```python
from build123d import *

# Parameters (mm, degrees)
F3_T     = -2.54
F5_D     = 7.62
F5_DEPTH = 38.101


# Not quite as in the source:
# - a feature of the source that left no trace in its solid (it failed there, or was rolled back) is left out


with BuildPart() as f1:
    # F0 (on Front) → F1 (revolve)
    with BuildSketch(Plane.XZ):
        Polygon((0, 0), (0, 63.5), (-38.1, 63.5), (-26.903236725, 0), align=None)
    revolve(axis=Axis((0, 0, 31.75), (0, 0, 1)))

    # F3
    f3_openings = [f1.faces().sort_by_distance(p)[0] for p in [
        (0, 0, 63.5),
    ]]
    offset(amount=F3_T, openings=f3_openings)

    # F5 (through all, one way)
    with BuildSketch(Plane.YZ):
        with Locations((0, 12.7)):
            Circle(F5_D / 2)
    extrude(amount=-F5_DEPTH, mode=Mode.SUBTRACT)


solid = f1.part
```
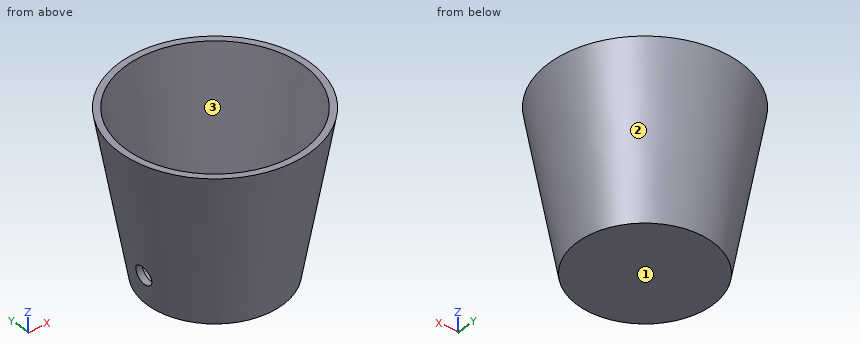
Here's how the part is built. I have some questions about the finished solid (model axes, mm). Face numbers are marked on the shaded views. Give positions to 0.01 mm unless a question says otherwise; leave off trailing zeros. Order: outer loops, then holes, each group sorted by start corner. A loop starts at its lowest first (then second) coordinate and runs counter-clockwise, first axis right, second up. Notation, with made-up numbers: (46, 62) - (61, 62) arc R7 ccw to (61, 70) - close; hole circle Ø11 at (53.25, -21.75). An arc over 180 degrees is marked (long way). Answer as a JSON object with one key per item and string values. Group by question number.
Item 1: If we section it at C-C on z = 21: Please give me the cut outline in (x, y).
Item 2: Please list where these lines run through material, in increasing order: probe 1 along Z at (x, y) = (-26.65, 0); probe 2 along Z at (x, y) = (-6, 2.5); probe 3 along Y at (x, z) = (24.5, 60.5).
Item 3: If we section it at B-B on z = 7.5: Please give me the cut outline in (x, y), and give its area (3 significant figures).
Item 4: If we mould it in two halves opening along X, with no side actions, what happens to the marked faces 1, 2 and 3? For each: pulls with the +X half, pulls with the -X half, needs draft (parallel to the pull), parting line crosses it, or undercut.
Item 5: For P1, Ø5, axis at y = -13, z = 26.5, coming from the +X side; P2, Ø12, axis at y = 5, z = 30, coming from the +X side; P3, Ø3, axis at x = -30.5, z = 39.5, coming from the +Y side, each with a flat end and sliding along its axis, tell me the tip position at first contact or that it passes through.
Item 6: If we section it at A-A on x = 0: Please give me the cut outline in (y, z), and give its area (3 significant figures).
Result set:
{
 "1": {"outline": "circle Ø61.21 at (0, 0); hole circle Ø56.05 at (0, 0)"},
 "2": {"probe 1": "0 to 8.89", "probe 2": "0 to 2.54", "probe 3": "-28.48 to -24.98, 24.98 to 28.48"},
 "3": {"outline": "circle Ø56.45 at (0, 0); hole circle Ø51.29 at (0, 0)", "area": "437 mm²"},
 "4": {"face 1": "needs draft", "face 2": "parting line crosses it", "face 3": "undercut"},
 "5": {"P1": "x = 29.89", "P2": "x = 33.06", "P3": "y = 17.55"},
 "6": {"outline": "(-38.1, 63.5) - (-26.9, 0) - (26.9, 0) - (38.1, 63.5) - (35.52, 63.5) - (24.77, 2.54) - (-24.77, 2.54) - (-35.52, 63.5) - close", "area": "452 mm²"}
}
